```python
from build123d import *

# Parameters (mm, degrees)
SKETCH_1_W                  = 47.7
SKETCH_1_H                  = 22.8
EXTRUDE_1_DEPTH             = 1
SKETCH_2_W                  = 1
SKETCH_2_H                  = 1
CUT_EXTRUDE_1_DEPTH         = 27.453402428
HOLE_WIZARD_1_0_1_1_D       = 1
HOLE_WIZARD_2_4_2_4_1_D     = 2.4
HOLE_WIZARD_2_4_2_4_1_DEPTH = 14
FILLET_1_R                  = 1
FILLET_2_R                  = 2


with BuildPart() as part:
    # 草图1 → 凸台-拉伸1 (new body)
    with BuildSketch(Plane.XZ):
        Rectangle(SKETCH_1_W, SKETCH_1_H)
    extrude(amount=-EXTRUDE_1_DEPTH)

    # 草图2 → 切除-拉伸1 (cut, through all)
    with BuildSketch(Plane(origin=(0, 1, 0), x_dir=(-1, 0, 0), z_dir=(0, 1, 0))):
        with Locations((3.55, 9.9)):
            Rectangle(SKETCH_2_W, SKETCH_2_H)
    extrude(amount=-CUT_EXTRUDE_1_DEPTH, mode=Mode.SUBTRACT)

    # 草图3 → 旋转1 (revolve)
    with BuildSketch(Plane(origin=(0, 0, 0), x_dir=(-1, 0, 0), z_dir=(0, 0, -1)), mode=Mode.PRIVATE) as revolve_1_sk:
        with BuildLine():
            Line((-21, 1), (-13, 1))
            Line((-13, 1), (-13, 14))
            Line((-13, 14), (-20.5, 14))
            Line((-20.5, 14), (-20.5, 11))
            ThreePointArc((-20.5, 11), (-20.853553391, 10.853553391), (-21, 10.5))
            Line((-21, 10.5), (-21, 1))
        make_face()
    revolve(revolve_1_sk.sketch.rotate(Axis((13, 1, 0), (0, 1, 0)), 270), axis=Axis((13, 1, 0), (0, 1, 0)))

    # 草图4 → 旋转2 (revolve)
    with BuildSketch(Plane(origin=(0, 0, 0), x_dir=(-1, 0, 0), z_dir=(0, 0, -1)), mode=Mode.PRIVATE) as revolve_2_sk:
        with BuildLine():
            Line((5, 1), (13, 1))
            Line((13, 1), (13, 14))
            Line((13, 14), (5.5, 14))
            Line((5.5, 14), (5.5, 11))
            ThreePointArc((5.5, 11), (5.146446609, 10.853553391), (5, 10.5))
            Line((5, 10.5), (5, 1))
        make_face()
    revolve(revolve_2_sk.sketch.rotate(Axis((-13, 1, 0), (0, 1, 0)), 270), axis=Axis((-13, 1, 0), (0, 1, 0)))

    # Ø1.0 (1) 直径孔1 (through all)
    with Locations(Plane(origin=(0, 1, 0), x_dir=(1, 0, 0), z_dir=(0, 1, 0))):
        with Locations((-0.55, -9.9), (1.95, -9.9), (4.45, -9.9), (-2.3, -8.4), (0, -8.4), (3.2, -8.4), (1.407287445, -8.4)):
            Hole(HOLE_WIZARD_1_0_1_1_D / 2)

    # Ø2.4 (2.4) 直径孔1
    with Locations(Plane(origin=(0, 0, 0), x_dir=(-1, 0, 0), z_dir=(0, -1, 0))):
        with Locations((21, 8.6), (-21, 8.6), (-21, -8.6), (21, -8.6)):
            Hole(HOLE_WIZARD_2_4_2_4_1_D / 2, depth=HOLE_WIZARD_2_4_2_4_1_DEPTH)

    # 圆角1
    fillet_1_edges = [part.edges().sort_by_distance(p)[0] for p in [
        (13, 14, -7.5),
        (-13, 14, -7.5),
    ]]
    fillet(fillet_1_edges, radius=FILLET_1_R)

    # 圆角2
    fillet_2_edges = [part.edges().sort_by_distance(p)[0] for p in [
        (-23.85, 0.5, 11.4),
        (23.85, 0.5, 11.4),
        (23.85, 0.5, -11.4),
        (-23.85, 0.5, -11.4),
    ]]
    fillet(fillet_2_edges, radius=FILLET_2_R)


solid = part.part
```
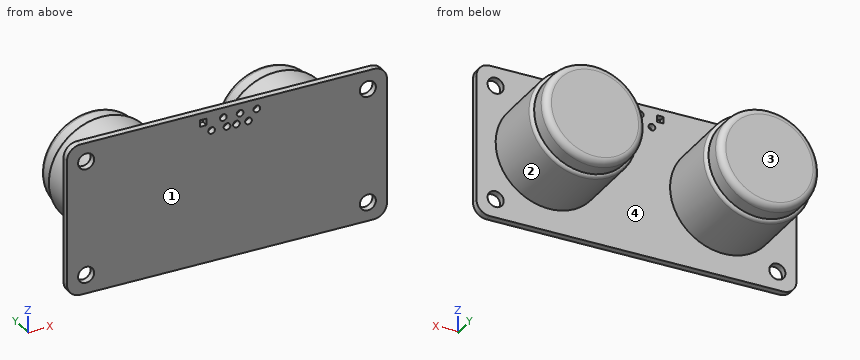
Part model, mm, in its own coordinate system. Face numbers are marked on the shaded views. A direction names the side the tool comes from. Round coordinates to 2 decimals unless told otherwise and drop trailing zeros. Loops run counter-clockwise (first coordinate to the right, second up) from the corner with the lowest first, then second, coordinate; pieces in that order, holes last. Notation, with made-up numbers: (44, 70.25) -> (93, 70.25) arc R26 cw to (93, 105.25) -> close; hole circle Ø1 at (69, 8.5). An arc over 180 degrees is marked (long way). Use one line per item in the form item = value. Start each with the question number.
Item 1: Band-saw the part on C-C (y = 2). List the corners of the cut face in (x, z).
Item 2: Two-plate mould, pull along X, no slides. Class the marked faces 3 and 4: released by +X, released by -X, zero draft, split by the parting line, or undercut.
Item 3: Band-saw the part on D-D (z = 0). List the corners of the cut face in (x, y), plus the area to 3 significant figures.
Item 4: Tool access for the marked faces 1 and 2: list every direction of +Z, -Z, +X, -X, +Y, -Y with a clear straight run to the whole face (end or side of a thin tool).
Item 5: Band-saw the part on B-B (x = 3.2). List the corners of the cut face in (y, z), plus the area to 3 significant figures.
Item 6: Drill centre lines: line 1 along Z through (x, y) = (21, 0.6); line 2 along X through (y, z) = (0.7, 9.9); line 3 along Z through (x, y) = (0, 0.7). Where is each one in solid material? Low to high.
Item 7: Drop flat-ended pins along their axis: pin 1 Ø1 at (x, z) = (-17, -1.5) entering from -Y; pin 2 Ø1 at (y, z) = (4.5, -6) entering from -X; pin 3 Ø1 at (x, z) = (0, -1.5) entering from +Y; pin 4 Ø0.8 at (y, z) = (0.5, 10) entering from -X. Give the stop position or say it passes through.
Item 8: Band-saw the part on A-A (z = -8.6). List the corners of the cut face in (x, y), plus the area to 3 significant figures.
Data:
q1.outline = circle Ø16 at (-13, 0); circle Ø16 at (13, 0)
q2.face_3 = zero draft
q2.face_4 = undercut
q3.outline = (-23.85, 0) -> (23.85, 0) -> (23.85, 1) -> (21, 1) -> (21, 10.5) arc R0.5 ccw to (20.5, 11) -> (20.5, 13) arc R1 ccw to (19.5, 14) -> (6.5, 14) arc R1 ccw to (5.5, 13) -> (5.5, 11) arc R0.5 ccw to (5, 10.5) -> (5, 1) -> (-5, 1) -> (-5, 10.5) arc R0.5 ccw to (-5.5, 11) -> (-5.5, 13) arc R1 ccw to (-6.5, 14) -> (-19.5, 14) arc R1 ccw to (-20.5, 13) -> (-20.5, 11) arc R0.5 ccw to (-21, 10.5) -> (-21, 1) -> (-23.85, 1) -> close
q3.area = 457 mm^2
q4.face_1 = +Z, -Z, +X, -X, -Y
q4.face_2 = +Y
q5.outline = (0, -11.4) -> (1, -11.4) -> (1, 7.9) -> (0, 7.9) -> close; (0, 8.9) -> (1, 8.9) -> (1, 11.4) -> (0, 11.4) -> close
q5.area = 21.8 mm^2
q6.line_1 = -11.4 to -9.8, -7.4 to 7.4, 9.8 to 11.4
q6.line_2 = -23.79 to -4.05, -3.05 to -1.05, -0.05 to 1.45, 2.45 to 3.95, 4.95 to 23.79
q6.line_3 = -11.4 to 7.9, 8.9 to 11.4
q7.pin_1 = 0
q7.pin_2 = -18.81
q7.pin_3 = 1
q7.pin_4 = -23.84
q8.outline = (-23.85, 0) -> (-22.2, 0) -> (-22.2, 1) -> (-23.85, 1) -> close; (-19.8, 0) -> (19.8, 0) -> (19.8, 1) -> (-19.8, 1) -> close; (22.2, 0) -> (23.85, 0) -> (23.85, 1) -> (22.2, 1) -> close
q8.area = 42.9 mm^2
